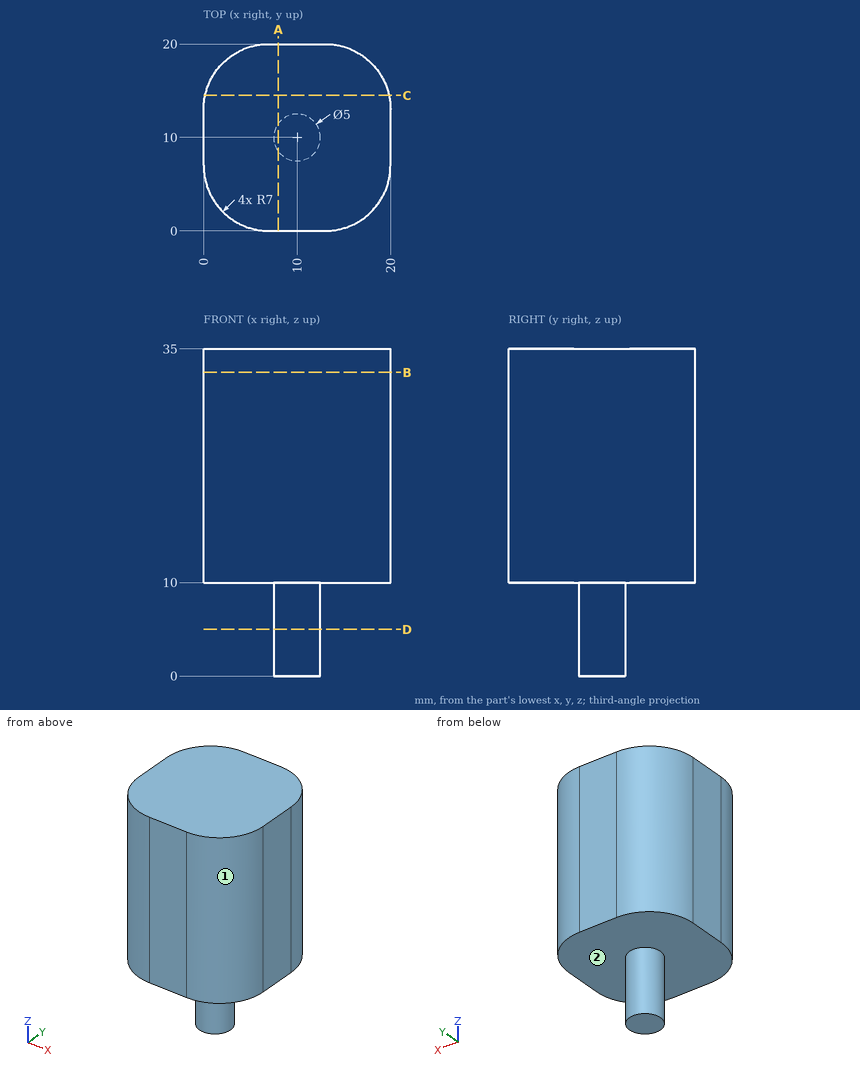
Part print with two shaded views. Sizes in mm from the minimum x, y, z corner. A direction names the side the tool comes from. Give positions to 0.01 mm unless a question says otherwise; leave off trailing zeros. Order: outer loops, then holes, each group sorted by start corner. A loop starts at its lowest first (then second) coordinate and runs counter-clockwise, first axis right, second up. Notation, with made-up numbers: M 34,22.25 L 72,22.25 A15 ccw 72,51.25 Z; hole C -15,-17 d5. An arc over 180 degrees is marked long. Write item = value, one per line.
Q1. Cut at A-A, the plane x = 8. List the corners of the cut face in (y, z), then the cut area to 3 significant figures.
Derived:
outline = M 0,10 L 8.5,10 L 8.5,0 L 11.5,0 L 11.5,10 L 20,10 L 20,35 L 0,35 Z
area = 530 mm2
Q2. Flat gauge pin, fed straight in: pin 1 (1.5 mm diameter, centred on x = 15.5, y = 5, fed in from -Z). Where does the tip first touch, or does it go through?
Derived:
pin_1 = 10
Q3. Drill centre lines: line 1 (Z direction, x = 4, y = 18.5); line 2 (Y direction, x = 14, z = 20.5); line 3 (X direction, y = 13.5, z = 24). Where is each one in solid material? Low to high. Write a range as [from, to].
Derived:
line_1 = [10, 35]
line_2 = [0.07, 19.93]
line_3 = [0.02, 19.98]
Q4. Cut at C-C, the plane y = 14.5. List the corners of the cut face in (x, z), then the cut area to 3 significant figures.
Derived:
outline = M 0.16,10 L 19.84,10 L 19.84,35 L 0.16,35 Z
area = 492 mm2
Q5. Tool access for the marked faces 1 and 2: list every direction of +Z, -Z, +X, -X, +Y, -Y with a clear straight run to the whole face (end or side of a thin tool).
Derived:
face_1 = +Z, -Z, +X, -Y
face_2 = -Z
Q6. Cut at D-D, the plane z = 5. List the corners of the cut face in (x, y).
Derived:
outline = C 10,10 d5
Q7. Cut at B-B, the plane z = 32.5. List the corners of the cut face in (x, y), then the cut area to 3 significant figures.
Derived:
outline = M 0,7 A7 ccw 7,0 L 13,0 A7 ccw 20,7 L 20,13 A7 ccw 13,20 L 7,20 A7 ccw 0,13 Z
area = 358 mm2
